```python
from build123d import *

# Parameters (mm, degrees)
F0_W     = 10
F0_H     = 7.5
F1_DEPTH = 20
F2_SIZE  = 2


with BuildPart() as f1:
    # F0 (on Front) → F1 (new body)
    with BuildSketch(Plane.XZ):
        Polygon((0, 30), (0, 0), (5, 0), (5, 12.5), (10, 12.5), (15, 0), (20, 0), (15, 12.5), (20, 12.5), (20, 30), align=None)
        with Locations((10, 21.25)):
            Rectangle(F0_W, F0_H, mode=Mode.SUBTRACT)
    extrude(amount=F1_DEPTH)

    # F2
    f2_edges = [f1.edges().sort_by_distance(p)[0] for p in [
        (20, -10, 30),
        (20, -10, 12.5),
        (5, -10, 17.5),
        (5, -10, 25),
        (5, -10, 12.5),
        (15, -10, 25),
        (15, -10, 17.5),
    ]]
    chamfer(f2_edges, length=F2_SIZE)


solid = f1.part
```
Part model, mm, in its own coordinate system. A direction names the side the tool comes from. Coordinates: 2 decimals unless noted, no trailing zeros. Loops run counter-clockwise (first coordinate to the right, second up) from the corner with the lowest first, then second, coordinate; pieces in that order, holes last. Notation, with made-up numbers: (37, 30.25) - (68, 30.25) arc R27 cw to (68, 48.25) - close; hole circle Ø9 at (2, 83.25). An arc over 180 degrees is marked (long way). Write item = value, one per line. Start each with the question number.
Item 1: Mould opens along X. For faces 1 (the flat face through (6, -10, 24)), 2 (the flat face through (17.535, -9.86, 6.163)), 3 (the flat face through (10, -20, 15)) say: released by +X, released by -X, zero draft, split by the parting line, or undercut.
Item 2: 3-axis set-ups, long thin cutter, end or side, ignore diameter. For faces 4 (the flat face through (12.465, -9.86, 6.337)), 5 (the flat face through (10, -10, 25)), 6 (the flat face through (16, -10, 12.5)), 7 (the flat face through (9, -10, 30)), 8 (the flat face through (0, -10, 15)): which of +Z, -Z, +X, -X, +Y, -Y reach the whole face in a straight line?
Item 3: Wall check: L1, parallel to X at y = -4, z = 20.75; L2, parallel to Z at x = 9.5, y = -13.5; L3, parallel to X at y = -2.75, z = 12. Give the ranges that are in metal, low to high. Write a range as from..to.
Item 4: Cut at A-A, the plane z = 19. Give the cut face in (x, y).
Item 5: Flat gauge pins, fed straight in: pin 1 Ø8.5 at (y, z) = (-12, 5.5) entering from +X; pin 2 Ø2.5 at (x, y) = (8, -13.5) entering from -Z; pin 3 Ø2 at (x, y) = (8.5, -5) entering from -Z. Where does each tip first touch, or does it go through?
Item 6: Cut at D-D, the plane z = 13.5. Give the cut face in (x, y), and give its area (3 significant figures).
Item 7: Cut at C-C, the plane y = -2.75. Give the cut face in (x, z), and give its area (3 significant figures).
Item 8: Cut at B-B, the plane x = 13.5. Give the cut face in (y, z).
The answers:
q1.face_1 = undercut
q1.face_2 = released by +X
q1.face_3 = zero draft
q2.face_4 = -Z, +Y, -Y
q2.face_5 = +Y, -Y
q2.face_6 = +X, +Y, -Y
q2.face_7 = +Z, +X, -X, +Y, -Y
q2.face_8 = +Z, -Z, -X, +Y, -Y
q3.L1 = 0..5, 15..20
q3.L2 = 12.5..17.5, 25..30
q3.L3 = 0..6.5, 10.2..15.2
q4.outline = (0, -20) - (5.5, -20) - (5.5, 0) - (0, 0) - close; (14.5, -20) - (20, -20) - (20, 0) - (14.5, 0) - close
q5.pin_1 = 19.5
q5.pin_2 = 12.25
q5.pin_3 = 12.5
q6.outline = (0, -20) - (19, -20) - (19, 0) - (0, 0) - close
q6.area = 380 mm2
q7.outline = (0, 0) - (5, 0) - (5, 10.5) - (7, 12.5) - (10, 12.5) - (15, 0) - (20, 0) - (15, 12.5) - (18, 12.5) - (20, 14.5) - (20, 28) - (18, 30) - (0, 30) - close; hole (5, 19.5) - (7, 17.5) - (13, 17.5) - (15, 19.5) - (15, 23) - (13, 25) - (7, 25) - (5, 23) - close
q7.area = 406 mm2
q8.outline = (-20, 3.75) - (0, 3.75) - (0, 18) - (-20, 18) - close; (-20, 24.5) - (0, 24.5) - (0, 30) - (-20, 30) - close
